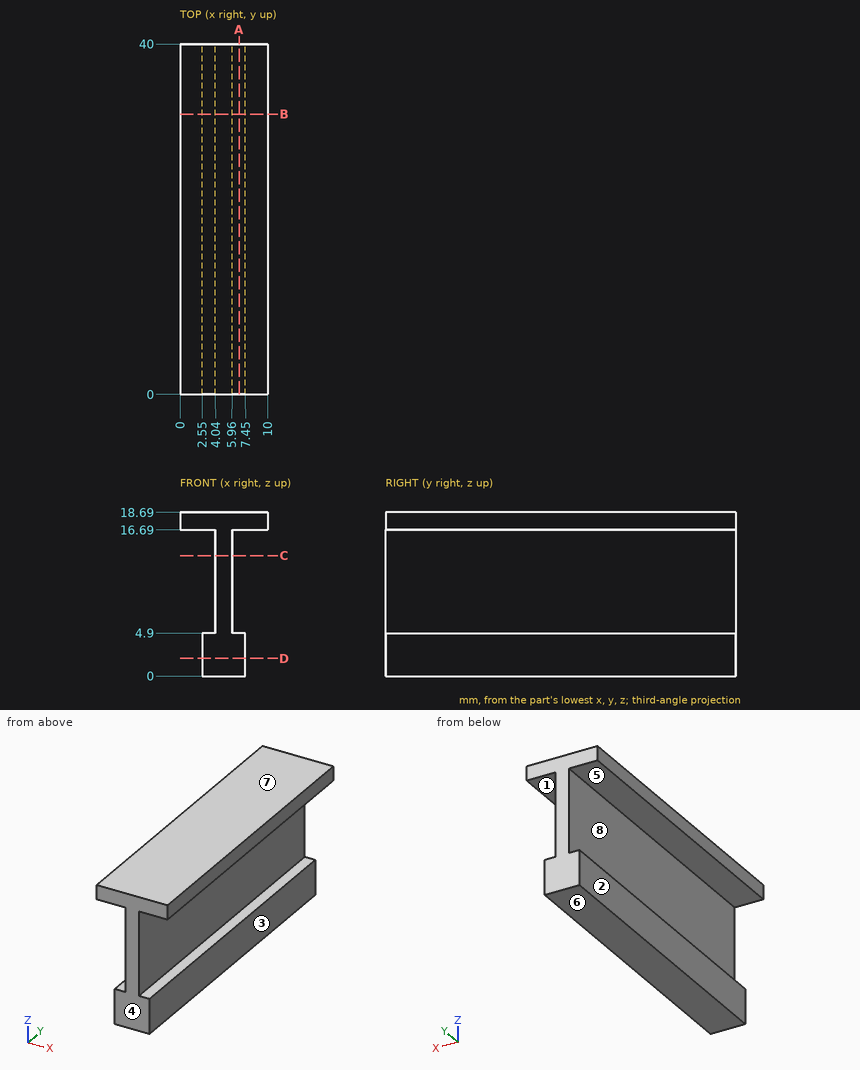
Could you check a few things on this drawing? It's one solid part, dimensions in mm from its lowest x, y, z. A direction names the side the tool comes from. Coordinates: 2 decimals unless noted, no trailing zeros. Loops run counter-clockwise (first coordinate to the right, second up) from the corner with the lowest first, then second, coordinate; pieces in that order, holes last. Notation, with made-up numbers: (57.5, 21) - (80.5, 21) arc R15 ccw to (80.5, 41) - close; hole circle Ø6 at (35, -21). An arc over 180 degrees is marked (long way). Return JSON: item names as keys, results as strings. Group by question number.
Item 1: If we section it at D-D on z = 2: Write out the boundary of the cut face in (x, y), and give its area (3 significant figures).
Item 2: If we section it at B-B on y = 32: Write out the boundary of the cut face in (x, z).
Item 3: If we section it at A-A on x = 6.75: Write out the boundary of the cut face in (y, z).
Item 4: I need wall thicknesses on line 1 (Z direction, x = 4, y = 35); line 2 (X direction, y = 4, z = 10.5); line 3 (Z direction, x = 1.75, y = 22). Which ranges of each line are inside material? Lowest first, please. Write a range as from..to.
Item 5: On a 3-axis mill with a long thin cutter (end or side, diameter ignored), from which of +Z, -Z, +X, -X, +Y, -Y can I reach the whole of each face in a straight line? I mean the marked faces 1, 2, 3, 4 and 5. Say none if no direction works.
Item 6: Will these pins go through, and if not, where does the flat tip stop? P1, Ø1.5, axis at y = 19.5, z = 3.5, coming from the +X side; P2, Ø3, axis at y = 20, z = 11.5, coming from the +X side; P3, Ø6, axis at x = 2, z = 7.5, coming from the -Y side; P4, Ø2.5, axis at y = 13.5, z = 3, coming from the -X side.
Item 7: If we section it at C-C on z = 13.75: Write out the boundary of the cut face in (x, y), and give its area (3 significant figures).
Item 8: We'd pull the mould along Z, two halves only. Please class the marked faces 6, 7 and 8: +Z half, -Z half, draft (parallel to the pull), parting line (faces both ways), or undercut.
Calculated:
{
 "1": {"outline": "(2.55, 0) - (7.45, 0) - (7.45, 40) - (2.55, 40) - close", "area": "196 mm^2"},
 "2": {"outline": "(0, 16.69) - (4.04, 16.69) - (4.04, 4.9) - (2.55, 4.9) - (2.55, 0) - (7.45, 0) - (7.45, 4.9) - (5.96, 4.9) - (5.96, 16.69) - (10, 16.69) - (10, 18.69) - (0, 18.69) - close"},
 "3": {"outline": "(0, 0) - (40, 0) - (40, 4.9) - (0, 4.9) - close; (0, 16.69) - (40, 16.69) - (40, 18.69) - (0, 18.69) - close"},
 "4": {"line 1": "z = 0..4.9, 16.69..18.69", "line 2": "x = 4.04..5.96", "line 3": "z = 16.69..18.69"},
 "5": {"face 1": "+X, +Y, -Y", "face 2": "-Z, -X, +Y, -Y", "face 3": "-Z, +X, +Y, -Y", "face 4": "+Z, -Z, +X, -X, -Y", "face 5": "-X, +Y, -Y"},
 "6": {"P1": "stops at x = 7.45", "P2": "stops at x = 5.96", "P3": "stops at y = 0", "P4": "stops at x = 2.55"},
 "7": {"outline": "(4.04, 0) - (5.96, 0) - (5.96, 40) - (4.04, 40) - close", "area": "76.8 mm^2"},
 "8": {"face 6": "-Z half", "face 7": "+Z half", "face 8": "undercut"}
}
